from build123d import *

# Parameters (mm, degrees)
F0_R     = 8.464637
F1_DEPTH = 2
F2_R     = 2
F3_D     = 2


with BuildPart() as f1:
    # F0 (on Top) → F1 (new body)
    with BuildSketch(Plane.XY):
        Polygon((17.556544, -28.5), (35.5, -28.5), (35.5, 28.5), (-35.5, 28.5), (-35.5, -28.5), (-17.556544, -28.5), (-11.704362, -17.429322), (0, -17.429322), (11.704362, -17.429322), align=None)
        with Locations((-12.535542, 0.055034)):
            Circle(F0_R, mode=Mode.SUBTRACT)
        with Locations((12.535542, 0.055034)):
            Circle(F0_R, mode=Mode.SUBTRACT)
    extrude(amount=F1_DEPTH)

    # F2
    f2_edges = [f1.edges().sort_by_distance(p)[0] for p in [
        (-35.5, 28.5, 1),
        (-35.5, -28.5, 1),
        (-17.556544, -28.5, 1),
        (-11.704362, -17.429322, 1),
        (11.704362, -17.429322, 1),
        (17.556544, -28.5, 1),
        (35.5, -28.5, 1),
        (35.5, 28.5, 1),
    ]]
    fillet(f2_edges, radius=F2_R)

    # F3 (through all)
    with Locations(Plane(origin=(0, 0, 0), x_dir=(1, 0, 0), z_dir=(0, 0, -1))):
        with Locations((-29.769791, 22.849604), (29.769791, 22.849604), (29.769791, -22.849604), (-29.769791, -22.849604)):
            Hole(F3_D / 2)


solid = f1.part
Source: CAD feature listing. Evaluate the final solid. Frame: model axes, mm. A direction names the side the tool comes from. Round coordinates to 2 decimals unless told otherwise and drop trailing zeros. Write each loop counter-clockwise with the first axis right and the second up, starting at its lowest first coordinate (ties: lowest second). Pieces come first, ordered by that corner, then holes. Notation, with made-up numbers: (20, 54.25) - (42, 54.25) arc R17 cw to (42, 70.25) - close; hole circle Ø1 at (76, 47). An arc over 180 degrees is marked (long way). Use CSV: the item, a comma, the result in double quotes. Start each with the question number.
(1) Cut plane A-A, the plane y = -6. Return loops of the section in (x, z).
(2) Material intervals for probe 1 along X at (y, z) = (-0.5, 1.4); probe 2 along X at (y, z) = (-1, 1); probe 3 along Y at (x, z) = (-18, 0.5), sorted ascending. Write a range as [from, to].
(3) Set-up query: faces 1 (the face through (35.5, 0, 1)), 2 (the face through (17.74, -28.22, 1.01)). Return all of +Z, -Z, +X, -X, +Y, -Y with unobstructed straight access to the full face (end or side cutting, diameter ignored); none if empty.
(4) First-contact query: pin 1 Ø4 at (x, y) = (-1.5, -16.5) entering from -Z; pin 2 Ø15 at (x, y) = (12.54, 0.06) entering from +Z. Flat tips, straight axial feed; report the tip coordinate or a pass-through.
(5) Cut plane B-B, the plane x = 6. Return loops of the section in (y, z).
(6) Cut plane D-D, the plane y = 6. Return loops of the section in (x, z), and give its area (3 significant figures).
(7) Cut plane C-C, the plane z = 1.55. Return loops of the section in (x, y).
(8) Mould query, pull axis Y, two halves, no side actions, for faces 3 (the face through (-4.462, 2.598, 0.986)), 4 (the face through (0, 28.5, 1)), 5 (the face through (14.597, -22.902, 0.986)), 6 (the face through (0, 0, 2)). Classes: pulls with the +Y half, pulls with the -Y half, needs draft (parallel to the pull), parting line crosses it, or undercut.
Geometry says:
1,outline,"(-35.5, 0) - (-18.45, 0) - (-18.45, 2) - (-35.5, 2) - close; (-6.62, 0) - (6.62, 0) - (6.62, 2) - (-6.62, 2) - close; (18.45, 0) - (35.5, 0) - (35.5, 2) - (18.45, 2) - close"
2,probe 1,"[-35.5, -20.98], [-4.09, 4.09], [20.98, 35.5]"
2,probe 2,"[-35.5, -20.93], [-4.14, 4.14], [20.93, 35.5]"
2,probe 3,"[-28.35, -6.41], [6.52, 28.5]"
3,face 1,"+Z, -Z, +X, +Y, -Y"
3,face 2,"+Z, -Z, -Y"
4,pin 1,"z = 0"
4,pin 2,"through"
5,outline,"(-17.43, 0) - (-5.32, 0) - (-5.32, 2) - (-17.43, 2) - close; (5.43, 0) - (28.5, 0) - (28.5, 2) - (5.43, 2) - close"
6,outline,"(-35.5, 0) - (-18.56, 0) - (-18.56, 2) - (-35.5, 2) - close; (-6.51, 0) - (6.51, 0) - (6.51, 2) - (-6.51, 2) - close; (18.56, 0) - (35.5, 0) - (35.5, 2) - (18.56, 2) - close"
6,area,"93.8 mm²"
7,outline,"(-35.5, -26.5) arc R2 ccw to (-33.5, -28.5) - (-18.76, -28.5) arc R2 ccw to (-16.99, -27.43) - (-12.27, -18.49) arc R2 cw to (-10.5, -17.43) - (10.5, -17.43) arc R2 cw to (12.27, -18.49) - (16.99, -27.43) arc R2 ccw to (18.76, -28.5) - (33.5, -28.5) arc R2 ccw to (35.5, -26.5) - (35.5, 26.5) arc R2 ccw to (33.5, 28.5) - (-33.5, 28.5) arc R2 ccw to (-35.5, 26.5) - close; hole circle Ø2 at (-29.77, -22.85); hole circle Ø2 at (-29.77, 22.85); hole circle Ø16.93 at (-12.54, 0.06); hole circle Ø16.93 at (12.54, 0.06); hole circle Ø2 at (29.77, -22.85); hole circle Ø2 at (29.77, 22.85)"
8,face 3,"undercut"
8,face 4,"pulls with the +Y half"
8,face 5,"pulls with the -Y half"
8,face 6,"needs draft"
